from build123d import *

# Parameters (mm, degrees)
SKETCH_2_W                  = 1
SKETCH_2_H                  = 57.5
EXTRUDE_2_DEPTH             = 8
EXTRUDE_3_DEPTH             = 23
EXTRUDE_3_DEPTH_BACK        = 2
SKETCH_3_W                  = 21
SKETCH_3_H                  = 82
SKETCH_4_R                  = 4
EXTRUDE_4_DEPTH             = 20
SKETCH_5_R                  = 4
CUT_EXTRUDE_1_DEPTH         = 4.5
CUT_EXTRUDE_START           = -4.5
SKETCH_6_R                  = 4
CUT_EXTRUDE_2_DEPTH         = 4.5
HOLE_WIZARD_M51_AT_2_COUNT  = 2
HOLE_WIZARD_M51_AT_2_PITCH  = 68
CUT_EXTRUDE_3_DEPTH         = 0.6
HOLE_WIZARD_M41_D           = 3.3
HOLE_WIZARD_M41_DEPTH       = 6.5
HOLE_WIZARD_M41_CSINK_D     = 4.1
HOLE_WIZARD_M41_CSINK_ANGLE = 90
HOLE_WIZARD_M41_TIP         = 0.991420021
SKETCH_12_W                 = 16.5
SKETCH_12_H                 = 51
CUT_EXTRUDE_4_DEPTH         = 1.5
CHAMFER_1_SIZE              = 1.5


with BuildPart() as part:
    # Эскиз2 → Бобышка-Вытянуть2 (new body)
    with BuildSketch(Plane(origin=(0, 0, 3), x_dir=(-1, 0, 0), z_dir=(0, 0, -1))):
        Rectangle(SKETCH_2_W, SKETCH_2_H)
    extrude(amount=EXTRUDE_2_DEPTH)

    # Эскиз3 → Бобышка-Вытянуть3 (add, two sides: drawn at the far end of the back side and taken through both)
    with BuildSketch(Plane.XY.offset(3).offset(-EXTRUDE_3_DEPTH_BACK)):
        Rectangle(SKETCH_3_W, SKETCH_3_H)
    extrude(amount=EXTRUDE_3_DEPTH + EXTRUDE_3_DEPTH_BACK)

    # Эскиз4 → Бобышка-Вытянуть4 (add)
    with BuildSketch(Plane(origin=(0, 41, 0), x_dir=(1, 0, 0), z_dir=(0, 1, 0))):
        with Locations(Location((0, -13.5, 0), (0, 0, 270))):
            Circle(SKETCH_4_R)
    extrude(amount=EXTRUDE_4_DEPTH)

    # Эскиз5 → Вырез-Вытянуть1 (cut)
    with BuildSketch(Plane.ZY.offset(10.5)):
        with Locations((16, 34)):
            Circle(SKETCH_5_R)
        with Locations(Location((16, -34, 0), (0, 0, 180))):
            Circle(SKETCH_5_R)
    extrude(amount=-CUT_EXTRUDE_1_DEPTH, mode=Mode.SUBTRACT)

    # Эскиз6 → Вырез-Вытянуть2 (cut)
    with BuildSketch(Plane(origin=(10.5, 0, 0), x_dir=(0, 0, -1), z_dir=(1, 0, 0)).offset(CUT_EXTRUDE_START)):
        with Locations(Location((-16, 34, 0), (0, 0, 180))):
            Circle(SKETCH_6_R)
        with Locations((-16, -34)):
            Circle(SKETCH_6_R)
    extrude(amount=CUT_EXTRUDE_2_DEPTH, mode=Mode.SUBTRACT)

    # Эскиз8 → Отверстие обработанное метчиком M51 (revolve, cut)
    with BuildSketch(Plane(origin=(6, 34, 16), x_dir=(0, 0, -1), z_dir=(0, 1, 0))):
        Polygon((0, 0), (0, 12), (2.9, 12), (2.1, 11.2), (2.1, 0.8), (2.9, 0), align=None)
    hole_wizard_m51 = revolve(axis=Axis((12.35, 34, 16), (-1, 0, 0)), mode=Mode.SUBTRACT)

    # Отверстие обработанное метчиком M51 at 2: Отверстие обработанное метчиком M51 ×2
    with Locations(*[(0, -i * HOLE_WIZARD_M51_AT_2_PITCH, 0) for i in range(1, HOLE_WIZARD_M51_AT_2_COUNT)]):
        add(hole_wizard_m51, mode=Mode.SUBTRACT)

    # Эскиз9 → Вырез-Вытянуть3 (cut)
    with BuildSketch(Plane.XY.offset(26)):
        with BuildLine():
            Line((-4.75, 31.75), (-4.75, 41))
            Line((-4.75, 41), (-10.5, 41))
            Line((-10.5, 41), (-10.5, -41))
            Line((-10.5, -41), (-4.75, -41))
            Line((-4.75, -41), (-4.75, -31.75))
            ThreePointArc((-4.75, -31.75), (0, -27), (4.75, -31.75))
            Line((4.75, -31.75), (4.75, -41))
            Line((4.75, -41), (10.5, -41))
            Line((10.5, -41), (10.5, 41))
            Line((10.5, 41), (4.75, 41))
            Line((4.75, 41), (4.75, 31.75))
            ThreePointArc((4.75, 31.75), (0, 27), (-4.75, 31.75))
        make_face()
    extrude(amount=-CUT_EXTRUDE_3_DEPTH, mode=Mode.SUBTRACT)

    # Отверстие обработанное метчиком M41
    with Locations(Plane.XY.offset(26)):
        with Locations((0, 38.2), (0, 34), (0, -34), (0, -38.2)):
            CounterSinkHole(HOLE_WIZARD_M41_D / 2, HOLE_WIZARD_M41_CSINK_D / 2, depth=HOLE_WIZARD_M41_DEPTH, counter_sink_angle=HOLE_WIZARD_M41_CSINK_ANGLE)
            with Locations((0, 0, -(HOLE_WIZARD_M41_DEPTH + HOLE_WIZARD_M41_TIP / 2))):  # 118° drill point
                Cone(0, HOLE_WIZARD_M41_D / 2, HOLE_WIZARD_M41_TIP, mode=Mode.SUBTRACT)

    # Эскиз12 → Вырез-Вытянуть4 (cut)
    with BuildSketch(Plane.ZY.offset(10.5)):
        Polygon((2, 0), (4, 0.932615316), (4, -0.932615316), align=None)
        with Locations((13.25, 0)):
            Rectangle(SKETCH_12_W, SKETCH_12_H)
    extrude(amount=-CUT_EXTRUDE_4_DEPTH, mode=Mode.SUBTRACT)

    # Фаска1
    chamfer_1_edges = [part.edges().sort_by_distance(p)[0] for p in [
        (-9, -25.5, 13.25),
        (-9, 0, 5),
        (-9, 25.5, 13.25),
        (-9, 0, 21.5),
    ]]
    chamfer(chamfer_1_edges, length=CHAMFER_1_SIZE - 0.0001)  # a hair under: the kernel refuses the full size


solid = part.part
Can you work these out from the model? Positions are in its coordinate system, mm. A direction names the side the tool comes from. Give positions to 0.01 mm unless a question says otherwise; leave off trailing zeros. Write each loop counter-clockwise with the first axis right and the second up, starting at its lowest first coordinate (ties: lowest second). Pieces come first, ordered by that corner, then holes. Notation, with made-up numbers: M 41,54 L 93,54 A20 cw 93,85 Z; hole C 46.5,-5 d7. An arc over 180 degrees is marked long. Answer in a Markdown table with one row per item. Add a question column.
Item 1: On a 3-axis mill with a long thin cutter (end or side, diameter ignored), from which of +Z, -Z, +X, -X, +Y, -Y can I reach the whole of each face in a straight line? I mean faces 1 (the flat face through (-5, 41, 13)), 2 (the cylindrical face through (8.218, -30.034, 16.521)), 3 (the flat face through (-9, 0, 13)), 4 (the cylindrical face through (-0.89, -36.81, 22.51)). Say none if no direction works.
Item 2: For pin 1 Ø6.5 at (y, z) = (34, 16) entering from -X; pin 2 Ø3 at (y, z) = (5, -1.5) entering from +X; pin 3 Ø1.5 at (x, y) = (-8.5, -26) entering from -Z, each with a flat end and sliding along its axis, tell me the tip position at first contact or that it passes through.
Item 3: Imagine slicing it at D-D, the plane y = 43. Write out the boundary of the cut face in (x, z).
Item 4: We'd pull the mould along Y, two halves only. Please class faces 5 (the flat face through (0.5, 0, -2)), 6 (the flat face through (0, 61, 13)), 7 (the conical face through (0.1, 33.7, 18.7)): released by +Y, released by -Y, zero draft, split by the parting line, or undercut.
Item 5: Please list where these lines run through material, in increasing order: L1, parallel to Y at x = 2.25, z = 15.5; L2, parallel to Y at x = 0, z = 23.5; L3, parallel to Y at x = 5.5, z = 17.
Item 6: Imagine slicing it at A-A, the plane x = -7.25. Write out the boundary of the cut face in (y, z), plus the area to 3 significant figures.
Evaluation:
| question | item | result |
|---|---|---|
| 1 | face 1 | +Y |
| 1 | face 2 | +X |
| 1 | face 3 | -X |
| 1 | face 4 | +Z |
| 2 | pin 1 | stops at x = -6 |
| 2 | pin 2 | stops at x = 0.5 |
| 2 | pin 3 | stops at z = 1 |
| 3 | outline | C 0,13.5 d8 |
| 4 | face 5 | zero draft |
| 4 | face 6 | released by +Y |
| 4 | face 7 | undercut |
| 5 | L1 | y = -41 to -36.04, -31.96 to 31.96, 36.04 to 61 |
| 5 | L2 | y = -41 to -39.85, -36.55 to -35.65, -32.35 to 32.35, 35.65 to 36.55, 39.85 to 41 |
| 5 | L3 | y = -41 to -36.18, -31.82 to 31.82, 36.18 to 41 |
| 6 | outline | M -41,1 L 41,1 L 41,25.4 L -41,25.4 Z; hole C -34,16 d8; hole C 34,16 d8 |
| 6 | area | 1,900 mm² |
